```python
from build123d import *
from build123d.topology import SkipClean

# Parameters (mm, degrees)
EXTRUDE_1_DEPTH     = 1
SKETCH_2_R          = 13.5
EXTRUDE_2_DEPTH     = 12
FILLET_1_R          = 5
SKETCH_5_R          = 2
CUT_EXTRUDE_1_DEPTH = 33.53459697


with BuildPart() as part:
    # 草图1 → 凸台-拉伸1 (new body)
    with BuildSketch(Plane(origin=(0, 0, 0), x_dir=(1, 0, 0), z_dir=(0, 1, 0))):
        with BuildLine():
            Line((-20.071428571, 5.421047417), (-5.785714286, 12.197356689))
            ThreePointArc((-5.785714286, 12.197356689), (0, 13.5), (5.785714286, 12.197356689))
            Line((5.785714286, 12.197356689), (20.071428571, 5.421047417))
            ThreePointArc((20.071428571, 5.421047417), (23.5, 0), (20.071428571, -5.421047417))
            Line((20.071428571, -5.421047417), (5.785714286, -12.197356689))
            ThreePointArc((5.785714286, -12.197356689), (0, -13.5), (-5.785714286, -12.197356689))
            Line((-5.785714286, -12.197356689), (-20.071428571, -5.421047417))
            ThreePointArc((-20.071428571, -5.421047417), (-23.5, 0), (-20.071428571, 5.421047417))
        make_face()
    extrude(amount=EXTRUDE_1_DEPTH)

    # 草图2 → 凸台-拉伸2 (add)
    with SkipClean():  # the faces are left unmerged after this step: merging them gives an invalid solid
        with BuildSketch(Plane(origin=(0, 1, 0), x_dir=(1, 0, 0), z_dir=(0, 1, 0))):
            with Locations(Location((0, 0, 0), (0, 0, 115.376933525))):
                Circle(SKETCH_2_R)
        extrude(amount=EXTRUDE_2_DEPTH)

    # 草图4 → 旋转1 (revolve)
    with SkipClean():  # the faces are left unmerged after this step: merging them gives an invalid solid
        with BuildSketch(Plane(origin=(0, 0, 0), x_dir=(0, 0, -1), z_dir=(1, 0, 0))):
            with BuildLine():
                Line((0, 18), (0, 2))
                ThreePointArc((0, 2), (-8, 10), (0, 18))
            make_face()
        revolve(axis=Axis((0, 18, 0), (0, -1, 0)))

    # 圆角1
    fillet_1_edges = [part.edges().sort_by_distance(p)[0] for p in [
        (5.785714286, 13, 12.197356689),
    ]]
    fillet(fillet_1_edges, radius=FILLET_1_R)

    # 草图5 → 切除-拉伸1 (cut, through all)
    with SkipClean():  # the faces are left unmerged after this step: merging them gives an invalid solid
        with BuildSketch(Plane.XZ):
            with Locations(Location((-17.5, 0, 0), (0, 0, 270))):
                Circle(SKETCH_5_R)
            with Locations(Location((17.5, 0, 0), (0, 0, 270))):
                Circle(SKETCH_5_R)
        extrude(amount=-CUT_EXTRUDE_1_DEPTH, mode=Mode.SUBTRACT)


solid = part.part
```
The listing builds one solid part. Answer for the finished solid, in the listing's coordinates (mm). A direction names the side the tool comes from. Give positions to 0.01 mm unless a question says otherwise; leave off trailing zeros. Write each loop counter-clockwise with the first axis right and the second up, starting at its lowest first coordinate (ties: lowest second). Pieces come first, ordered by that corner, then holes. Notation, with made-up numbers: (-16.75, 67.5) -> (15.25, 67.5) arc R23 cw to (15.25, 76.5) -> close; hole circle Ø6 at (8.25, 57). An arc over 180 degrees is marked (long way). Use one line per item in the form item = value.
1) Section D-D on y = 1.75 is taken. Write down the section's boundary in (x, z), plus the area to 3 significant figures.
Result:
outline = circle Ø27 at (0, 0)
area = 573 mm²
2) Section B-B on x = -17.5 is taken. Write down the section's boundary in (y, z), plus the area to 3 significant figures.
Result:
outline = (0, -6.64) -> (1, -6.64) -> (1, -2) -> (0, -2) -> close; (0, 2) -> (1, 2) -> (1, 6.64) -> (0, 6.64) -> close
area = 9.28 mm²
3) Each of these flat-tipped pins is pushed along its axis until it touches: P1, Ø4, axis at y = 9.5, z = -0.5, coming from the -X side; P2, Ø1, axis at y = 5.5, z = 7.5, coming from the -X side; P3, Ø8.5, axis at x = 3, z = -3.5, coming from the +Y side; P4, Ø3, axis at x = -17.5, z = 0, coming from the +Y side. Where does it stop, or does it pass through?
Result:
P1 = -13.5
P2 = -11.54
P3 = 17.99
P4 = through
4) A tool of negligible diameter and unlimited length cuts with its end or side. For faces 1 (the flat face through (13.03, 0.49, 8.76)), 2 (the flat face through (-7, 13, 3)), from which of +Z, -Z, +X, -X, +Y, -Y can it reach the whole face along a straight path? Write none if from no direction.
Result:
face_1 = +Z, +X, +Y, -Y
face_2 = +Y
5) Straight lines are drawn through the part: probe 1 along Y at (x, z) = (-19, -2); probe 2 along X at (y, z) = (5, 9.5); probe 3 along Y at (x, z) = (6, -10). For each, find the intervals that lie inside material, in ascending order.
Result:
probe_1 = 0 to 1
probe_2 = -9.59 to 9.59
probe_3 = 0 to 11.87
6) Section A-A on z = 0 is taken. Write down the section's boundary in (x, y).
Result:
outline = (-23.5, 0) -> (-19.5, 0) -> (-19.5, 1) -> (-23.5, 1) -> close; (-15.5, 0) -> (15.5, 0) -> (15.5, 1) -> (13.5, 1) -> (13.5, 8) arc R5 ccw to (8.5, 13) -> (7.42, 13) arc R8 ccw to (-7.42, 13) -> (-8.5, 13) arc R5 ccw to (-13.5, 8) -> (-13.5, 1) -> (-15.5, 1) -> close; (19.5, 0) -> (23.5, 0) -> (23.5, 1) -> (19.5, 1) -> close
7) Section C-C on x = 0 is taken. Write down the section's boundary in (y, z), plus the area to 3 significant figures.
Result:
outline = (0, -13.5) -> (8, -13.5) arc R5 ccw to (13, -8.5) -> (13, -7.42) arc R8 ccw to (13, 7.42) -> (13, 8.5) arc R5 ccw to (8, 13.5) -> (0, 13.5) -> close
area = 394 mm²
8) For a pull along Z with two mould halves and no side action, classify faces 3 (the flat face through (-12.829, 0.493, 8.857)), 4 (the cylindrical face through (19.483, 0.493, 0.26)), 5 (the flat face through (12.829, 0.493, -8.857)), 6 (the cylindrical face through (-15.517, 0.493, 0.26)) as +Z half, -Z half, draft (parallel to the pull), parting line (faces both ways), or undercut.
Result:
face_3 = +Z half
face_4 = undercut
face_5 = -Z half
face_6 = undercut
